Check sheet for the modelled part. Datum: model origin and axes. Units: mm. Round coordinates to 2 decimals unless told otherwise and drop trailing zeros. Write each loop counter-clockwise with the first axis right and the second up, starting at its lowest first coordinate (ties: lowest second). Pieces come first, ordered by that corner, then holes.
Item 1: Go/stop test with flat-tipped pins: pin 1 Ø10 at (y, z) = (-9, 17.5) entering from +X; pin 2 Ø2 at (y, z) = (-4.5, 3) entering from +X; pin 3 Ø2 at (y, z) = (-15.5, -17) entering from +X. Record where each tip stops, or that it passes through.
Item 2: Material ranges on line 1 (Z direction, x = 6.5, y = -21.5); line 2 (X direction, y = -14, z = -21); line 3 (Z direction, x = -9.5, y = -18), recorded low to high.
Item 3: Cross-section at A-A on x = 0. Enter the section's corners in (y, z), plus the area to 3 significant figures.
Item 4: Release check for a two-part mould opening along X. For faces 1 (the cylindrical face through (-18.5, -12.3, -7.6)), 2 (the cylindrical face through (-0.34, -12.68, -1.55)), 3 (the flat face through (0, -25, -7)), 4 (the cylindrical face through (18.464, -12.325, -7.688)) record: +X half, -X half, draft (parallel to the pull), parting line (faces both ways), or undercut.
Item 5: Cross-section at B-B on x = -8. Enter the section's corners in (y, z).
from build123d import *

# Parameters (mm, degrees)
F1_DEPTH = 25
F2_R     = 1.5875
F3_DEPTH = 25


with BuildPart() as f1:
    # F0 (on Front) → F1 (new body)
    with BuildSketch(Plane.XZ):
        with BuildLine():
            Line((-17.3205080757, 10), (0, 0))
            Line((0, 0), (17.3205080757, 10))
            ThreePointArc((17.3205080757, 10), (0, 20), (-17.3205080757, 10))
        make_face()
        with BuildLine():
            ThreePointArc((21.6506350946, 12.5), (0, 25), (-21.6506350946, 12.5))
            Line((-21.6506350946, 12.5), (-17.3205080757, 10))
            ThreePointArc((-17.3205080757, 10), (0, 20), (17.3205080757, 10))
            Line((17.3205080757, 10), (21.6506350946, 12.5))
        make_face()
        with BuildLine():
            Line((19.3185165258, 5.1763809021), (24.1481456572, 6.4704761276))
            ThreePointArc((24.1481456572, 6.4704761276), (23.0969883128, 9.5670858091), (21.6506350946, 12.5))
            Line((21.6506350946, 12.5), (17.3205080757, 10))
            ThreePointArc((17.3205080757, 10), (18.4775906502, 7.6536686473), (19.3185165258, 5.1763809021))
        make_face()
        with BuildLine():
            Line((17.3205080757, 10), (0, 0))
            Line((0, 0), (19.3185165258, 5.1763809021))
            ThreePointArc((19.3185165258, 5.1763809021), (18.4775906502, 7.6536686473), (17.3205080757, 10))
        make_face()
        with BuildLine():
            Line((0, 0), (19.3185165258, -5.1763809021))
            ThreePointArc((19.3185165258, -5.1763809021), (19.8288972275, -2.6105238444), (20, 0))
            ThreePointArc((20, 0), (19.8288972275, 2.6105238444), (19.3185165258, 5.1763809021))
            Line((19.3185165258, 5.1763809021), (0, 0))
        make_face()
        with BuildLine():
            add(Edge.make_bspline(
                [(19.3185165258, -5.1763809021), (21.3890688866, 2.5510257083), (24.9246027925, 3.5726986487), (24.1481456572, 6.4704761276)],
                knots=[0, 0, 0, 0, 12.6085128471, 12.6085128471, 12.6085128471, 12.6085128471], degree=3))
            Line((24.1481456572, 6.4704761276), (19.3185165258, 5.1763809021))
            ThreePointArc((19.3185165258, 5.1763809021), (19.8288972275, 2.6105238444), (20, 0))
            ThreePointArc((20, 0), (19.8288972275, -2.6105238444), (19.3185165258, -5.1763809021))
        make_face()
        with BuildLine():
            Line((0, 0), (17.3205080757, -10))
            ThreePointArc((17.3205080757, -10), (18.4775906502, -7.6536686473), (19.3185165258, -5.1763809021))
            Line((19.3185165258, -5.1763809021), (0, 0))
        make_face()
        with BuildLine():
            ThreePointArc((-17.3205080757, -10), (0, -20), (17.3205080757, -10))
            Line((17.3205080757, -10), (0, 0))
            Line((0, 0), (-17.3205080757, 10))
            ThreePointArc((-17.3205080757, 10), (-19.8288972275, 2.6105238444), (-19.3185165258, -5.1763809021))
            ThreePointArc((-19.3185165258, -5.1763809021), (-18.4775906502, -7.6536686473), (-17.3205080757, -10))
        make_face()
        with BuildLine():
            Line((-10, -40), (10, -40))
            add(Edge.make_bspline(
                [(11.9704769274, -21.9478400334), (10.6395133933, -26.6376402025), (10, -32.1254718634), (10, -40)],
                knots=[14.6690901551, 14.6690901551, 14.6690901551, 14.6690901551, 30.8802499745, 30.8802499745, 30.8802499745, 30.8802499745], degree=3))
            ThreePointArc((11.9704769274, -21.9478400334), (0, -25), (-11.9704769274, -21.9478400334))
            add(Edge.make_bspline(
                [(-11.9704769274, -21.9478400334), (-10.6395133933, -26.6376402025), (-10, -32.1254718634), (-10, -40)],
                knots=[14.6690901551, 14.6690901551, 14.6690901551, 14.6690901551, 30.8802499745, 30.8802499745, 30.8802499745, 30.8802499745], degree=3))
        make_face()
        with BuildLine():
            ThreePointArc((-11.9704769274, -21.9478400334), (0, -25), (11.9704769274, -21.9478400334))
            add(Edge.make_bspline(
                [(17.3205080757, -10), (14.9453507879, -14.1138930984), (13.1748339439, -17.7041522123), (11.9704769274, -21.9478400334)],
                knots=[0, 0, 0, 0, 14.6690901551, 14.6690901551, 14.6690901551, 14.6690901551], degree=3))
            ThreePointArc((17.3205080757, -10), (0, -20), (-17.3205080757, -10))
            add(Edge.make_bspline(
                [(-17.3205080757, -10), (-14.9453507879, -14.1138930984), (-13.1748339439, -17.7041522123), (-11.9704769274, -21.9478400334)],
                knots=[0, 0, 0, 0, 14.6690901551, 14.6690901551, 14.6690901551, 14.6690901551], degree=3))
        make_face()
        with BuildLine():
            ThreePointArc((-21.6506350946, 12.5), (-23.0969883128, 9.5670858091), (-24.1481456572, 6.4704761276))
            add(Edge.make_bspline(
                [(-19.3185165258, -5.1763809021), (-21.3890688866, 2.5510257083), (-24.9246027925, 3.5726986487), (-24.1481456572, 6.4704761276)],
                knots=[0, 0, 0, 0, 12.6085128471, 12.6085128471, 12.6085128471, 12.6085128471], degree=3))
            ThreePointArc((-19.3185165258, -5.1763809021), (-19.8288972275, 2.6105238444), (-17.3205080757, 10))
            Line((-17.3205080757, 10), (-21.6506350946, 12.5))
        make_face()
    extrude(amount=F1_DEPTH)

    # F2 (on face) → F3 (cut)
    with BuildSketch(Plane.XZ.offset(25)):
        Circle(F2_R)
    extrude(amount=-F3_DEPTH, mode=Mode.SUBTRACT)


solid = f1.part
Response values:
1. pin 1: stops at x = 21.65
1. pin 2: stops at x = 23.77
1. pin 3: stops at x = 14.17
2. line 1: z = -40 to 24.14
2. line 2: x = -12.25 to 12.25
2. line 3: z = -40 to 23.12
3. outline: (-25, -40) - (0, -40) - (0, -1.59) - (-25, -1.59) - close; (-25, 1.59) - (0, 1.59) - (0, 25) - (-25, 25) - close
3. area: 1,550 mm2
4. face 1: -X half
4. face 2: undercut
4. face 3: draft
4. face 4: +X half
5. outline: (-25, -40) - (0, -40) - (0, 23.69) - (-25, 23.69) - close
